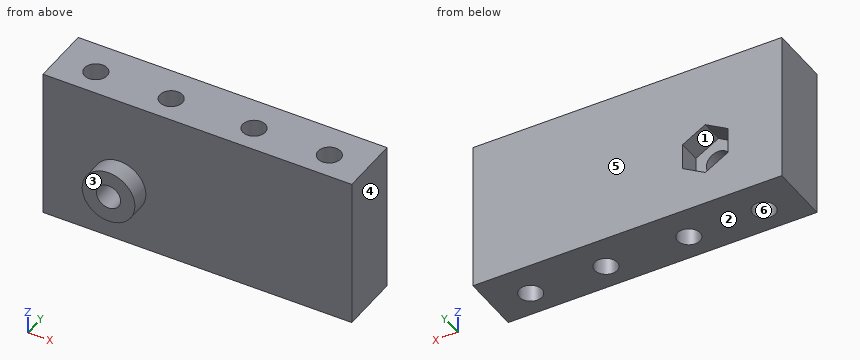
```python
from build123d import *

# Parameters (mm, degrees)
SKETCH1_W           = 41
SKETCH1_H           = 20
BOSS_EXTRUDE1_DEPTH = 8
SKETCH2_R           = 1.5
CUT_EXTRUDE1_DEPTH  = 47.314144708
LPATTERN1_COUNT     = 2
LPATTERN1_PITCH     = 10
LPATTERN2_COUNT     = 2
LPATTERN2_PITCH     = 21
LPATTERN3_COUNT     = 2
LPATTERN3_PITCH     = 31
SKETCH3_R           = 1.6
CUT_EXTRUDE6_DEPTH  = 47.314144708
BOSS_EXTRUDE6_START = 2.5
SKETCH13_R          = 3.5
SKETCH13_R_2        = 1.6
BOSS_EXTRUDE6_DEPTH = 2.5
CUT_EXTRUDE7_DEPTH  = 3


with BuildPart() as part:
    # Sketch1 → Boss-Extrude1 (new body)
    with BuildSketch(Plane(origin=(0, 0, 0), x_dir=(1, 0, 0), z_dir=(0, 1, 0))):
        with Locations((20.5, 10)):
            Rectangle(SKETCH1_W, SKETCH1_H)
    extrude(amount=BOSS_EXTRUDE1_DEPTH)

    # Sketch2 → Cut-Extrude1 (cut, through all)
    with BuildSketch(Plane.XY):
        with Locations((5, 3.455)):
            Circle(SKETCH2_R)
    cut_extrude1 = extrude(amount=-CUT_EXTRUDE1_DEPTH, mode=Mode.SUBTRACT)

    # LPattern1: Cut-Extrude1 ×2
    with Locations(*[(i * LPATTERN1_PITCH, 0, 0) for i in range(1, LPATTERN1_COUNT)]):
        add(cut_extrude1, mode=Mode.SUBTRACT)

    # LPattern2: Cut-Extrude1 ×2
    with Locations(*[(i * LPATTERN2_PITCH, 0, 0) for i in range(1, LPATTERN2_COUNT)]):
        add(cut_extrude1, mode=Mode.SUBTRACT)

    # LPattern3: Cut-Extrude1 ×2
    with Locations(*[(i * LPATTERN3_PITCH, 0, 0) for i in range(1, LPATTERN3_COUNT)]):
        add(cut_extrude1, mode=Mode.SUBTRACT)

    # Sketch3 → Cut-Extrude6 (cut, through all)
    with BuildSketch(Plane(origin=(0, 0, 0), x_dir=(1, 0, 0), z_dir=(0, 1, 0))):
        with Locations(Location((10.16, 12.135, 0), (0, 0, 90))):
            Circle(SKETCH3_R)
    extrude(amount=CUT_EXTRUDE6_DEPTH, mode=Mode.SUBTRACT)

    # Sketch13 → Boss-Extrude6 (add)
    with BuildSketch(Plane.XZ.offset(BOSS_EXTRUDE6_START)):
        with Locations(Location((10.16, -12.135, 0), (0, 0, 270))):
            Circle(SKETCH13_R)
        with Locations(Location((10.16, -12.135, 0), (0, 0, 270))):
            Circle(SKETCH13_R_2, mode=Mode.SUBTRACT)
    extrude(amount=-BOSS_EXTRUDE6_DEPTH)

    # Sketch14 → Cut-Extrude7 (cut)
    with BuildSketch(Plane(origin=(0, 8, 0), x_dir=(1, 0, 0), z_dir=(0, 1, 0))):
        Polygon((7.16, 10.402949192), (10.16, 8.670898385), (13.16, 10.402949192), (13.16, 13.867050808), (10.16, 15.599101615), (7.16, 13.867050808), align=None)
    extrude(amount=-CUT_EXTRUDE7_DEPTH, mode=Mode.SUBTRACT)


solid = part.part
```
Geometry check sheet. Reference: the model listing, model coordinates, mm. Face numbers are marked on the shaded views. A direction names the side the tool comes from. Give positions to 0.01 mm unless a question says otherwise; leave off trailing zeros. Order: outer loops, then holes, each group sorted by start corner. A loop starts at its lowest first (then second) coordinate and runs counter-clockwise, first axis right, second up.
1. Section check A-A, the plane y = 6.75. Enter the section's corners in (x, z).
2. Section check C-C, the plane z = -11.5. Enter the section's corners in (x, y) (3 decimals), and give its area (3 significant figures).
3. Section check B-B, the plane x = 26. Enter the section's corners in (y, z) (3 decimals).
4. Access from +Z, -Z, +X, -X, +Y, -Y to the whole of each face (thin tool, end or side, straight path). Record for the marked faces 1 and 2.
5. Section check D-D, the plane z = -17.5. Enter the section's corners in (x, y) (3 decimals).
6. Gauge pin test, flat ends, axial feed: pin 1 Ø1.8 at (x, z) = (10.5, -13.5) entering from +Y; pin 2 Ø1.5 at (x, z) = (32, -15) entering from -Y. Record the tip position at first contact, or that the pin passes through.
7. Release check for a two-part mould opening along Y. For the marked faces 3, 4, 5 and 6 record: pulls with the +Y half, pulls with the -Y half, needs draft (parallel to the pull), parting line crosses it, or undercut.
8. Thickness scan on L1, parallel to Y at x = 26, z = -13.5 (3 decimals); L2, parallel to X at y = 3.5, z = -4; L3, parallel to X at y = 4.75, z = -10.5. Record the ranges inside material, lowest first.
Values follow:
1. outline: (0, -20) - (41, -20) - (41, 0) - (0, 0) - close; hole (7.16, -13.87) - (10.16, -15.6) - (13.16, -13.87) - (13.16, -10.4) - (10.16, -8.67) - (7.16, -10.4) - close
2. outline: (0, 0) - (6.718, 0) - (6.718, -2.5) - (8.691, -2.5) - (8.691, 5) - (7.16, 5) - (7.16, 8) - (0, 8) - close; (11.629, -2.5) - (13.602, -2.5) - (13.602, 0) - (41, 0) - (41, 8) - (13.16, 8) - (13.16, 5) - (11.629, 5) - close; hole circle Ø3 at (5, 3.455); hole circle Ø3 at (15, 3.455); hole circle Ø3 at (26, 3.455); hole circle Ø3 at (36, 3.455)
2. area: 277 mm2
3. outline: (0, -20) - (1.955, -20) - (1.955, 0) - (0, 0) - close; (4.955, -20) - (8, -20) - (8, 0) - (4.955, 0) - close
4. face 1: +Y
4. face 2: -Z, +X, -X, +Y, -Y
5. outline: (0, 0) - (41, 0) - (41, 8) - (0, 8) - close; hole circle Ø3 at (5, 3.455); hole circle Ø3 at (15, 3.455); hole circle Ø3 at (26, 3.455); hole circle Ø3 at (36, 3.455)
6. pin 1: stops at y = 5
6. pin 2: stops at y = 0
7. face 3: pulls with the -Y half
7. face 4: needs draft
7. face 5: pulls with the +Y half
7. face 6: undercut
8. L1: y = 0 to 1.955, 4.955 to 8
8. L2: x = 0 to 3.5, 6.5 to 13.5, 16.5 to 24.5, 27.5 to 34.5, 37.5 to 41
8. L3: x = 0 to 4.24, 5.76 to 14.24, 15.76 to 25.24, 26.76 to 35.24, 36.76 to 41
